```python
from build123d import *

# Parameters (mm, degrees)
F1_DEPTH    = 10
F2_R        = 2.65
F2_R_2      = 2.7
F3_DEPTH    = 10.001
F4_T2_ANGLE = 34.0182957269
F6_DEPTH    = 6
F7_R        = 1.99999
F8_T1_DEPTH = 13.9199888123


# Not quite as in the source:
# - a fillet or chamfer that OpenCascade refuses, or shapes differently, is made with other operations: its cross-section is extruded or revolved along the edge and cut away or added
# - a fillet or chamfer is up to 0.001 mm smaller than in the source, because OpenCascade refuses the exact size


with BuildPart() as f1:
    # F0 (on Top) → F1 (new body)
    with BuildSketch(Plane.XY):
        with BuildLine():
            Line((-33.6606874732, -11.2477834763), (-53.6606874732, -11.1477834763))
            Line((-53.6606874732, -11.1477834763), (-53.7111874732, -21.2477834763))
            Line((-53.7111874732, -21.2477834763), (-41.7113374704, -21.3077827264))
            ThreePointArc((-41.7113374704, -21.3077827264), (-20.1551088941, -33.6039887965), (-10, -56.2477834763))
            Line((-10, -56.2477834763), (0, -56.2477834763))
            ThreePointArc((0, -56.2477834763), (0.8963967025, -47.7664020072), (1.3093095262, -39.2477834763))
            Line((1.3093095262, -39.2477834763), (1.0172378853, -32.2477834763))
            ThreePointArc((1.0172378853, -32.2477834763), (-3.5776423647, -21.3591536143), (-12.6606874732, -13.7978391557))
            Line((-12.6606874732, -13.7978391557), (-21.6606874732, -12.1477834763))
            ThreePointArc((-21.6606874732, -12.1477834763), (-27.6471372828, -11.5171142711), (-33.6606874732, -11.2477834763))
        make_face()
    extrude(amount=F1_DEPTH)

    # F2 (on face) → F3 (cut, through all)
    with BuildSketch(Plane.XY.offset(10)):
        with Locations((-46.6606874732, -17.1477834763)):
            Circle(F2_R)
        with Locations((-16.6606874732, -21.2477834763)):
            Circle(F2_R)
        with Locations((-6.6606874732, -50.2477834763)):
            Circle(F2_R)
        with Locations((-6.6606874732, -30.2477834763)):
            Circle(F2_R_2)
    extrude(amount=-F3_DEPTH, mode=Mode.SUBTRACT)

    # F4: fillet of radius 6 on 1 edges, made by hand

    # F4_s1 → F4_t2 (revolve, cut)
    with BuildSketch(Plane(origin=(-32.1356329931, -81.9445924317, 0), x_dir=(0, 0, 1), z_dir=(-0.3650924394, -0.9309712727, 0))):
        with BuildLine():
            ThreePointArc((0, -18.8349622687), (1.7573593129, -23.0776029558), (6, -24.8349622687))
            Line((6, -24.8349622687), (6, -24.9549622687))
            Line((6, -24.9549622687), (-0.12, -24.9549622687))
            Line((-0.12, -24.9549622687), (-0.12, -18.8349622687))
            Line((-0.12, -18.8349622687), (0, -18.8349622687))
        make_face()
    revolve(axis=Axis((-148.6606874732, -36.2477834763, 0), (0, 0, 1)), revolution_arc=F4_T2_ANGLE, mode=Mode.SUBTRACT)

    # F5 (on face) → F6 (join)
    with BuildSketch(Plane.XY):
        with BuildLine():
            ThreePointArc((-19.6606874732, -34.1590258202), (-19.1967513982, -34.6993177477), (-18.7425076385, -35.2477834763))
            Line((-18.7425076385, -35.2477834763), (-9.6606874732, -35.2477834763))
            Line((-9.6606874732, -35.2477834763), (-9.6606874732, -31.2477834763))
            Line((-9.6606874732, -31.2477834763), (-19.6606874732, -31.2477834763))
            Line((-19.6606874732, -31.2477834763), (-19.6606874732, -34.1590258202))
        make_face()
    extrude(amount=-F6_DEPTH)

    # F7 (radius 2 in the source; OpenCascade refuses exactly that, so slightly less here)
    f7_edges = [f1.edges().sort_by_distance(p)[0] for p in [
        (-19.660687, -31.247783, -3),
        (-9.660687, -31.247783, -3),
        (-9.660687, -35.247783, -3),
    ]]
    fillet(f7_edges, radius=F7_R)

    # F8: fillet of radius 7 on 1 edges, made by hand

    # F8_s2 → F8_t1 (cut)
    with BuildSketch(Plane.XY.offset(-13.9199888123)):
        with BuildLine():
            ThreePointArc((-15.5745121135, -35.2477834763), (-18.3484354275, -34.6747072699), (-20.6681674701, -33.0493118901))
            ThreePointArc((-20.6681674701, -33.0493118901), (-19.6852521083, -34.1309546714), (-18.7425076385, -35.2477834763))
            Line((-18.7425076385, -35.2477834763), (-15.5745121135, -35.2477834763))
        make_face()
    extrude(amount=F8_T1_DEPTH, mode=Mode.SUBTRACT)


solid = f1.part
```
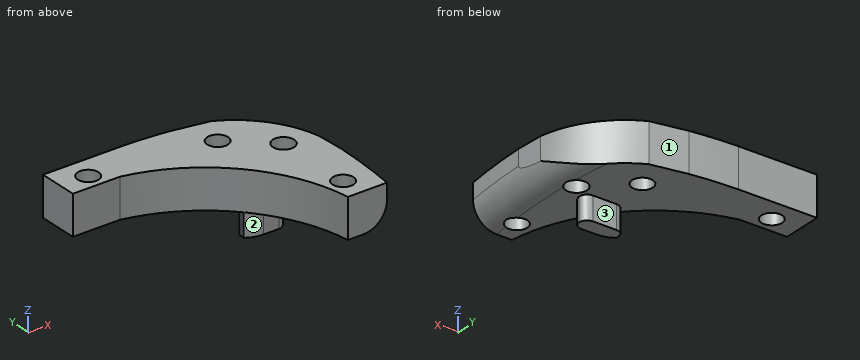
Source: CAD feature listing. Evaluate the final solid. Frame: model axes, mm. Face numbers are marked on the shaded views. A direction names the side the tool comes from. Round coordinates to 2 decimals unless told otherwise and drop trailing zeros. Write each loop counter-clockwise with the first axis right and the second up, starting at its lowest first coordinate (ties: lowest second). Pieces come first, ordered by that corner, then holes. Notation, with made-up numbers: M 36.5,-38.5 L 89.5,-38.5 A19 ccw 89.5,-23.5 Z; hole C 65.5,-29 d3. An arc over 180 degrees is marked long. Use CSV: the item, a comma, the result in double quotes. Start each with the question number.
Q1. Line query: line 1 (Z direction, x = -9, y = -36.5); line 2 (Y direction, x = -5, z = 1.5); line 3 (Y direction, x = -17, z = 1.25). Output: solid intervals per line, ascending. Write a range as from..to.
Q2. Cut plane C-C on x = -36. Output: boundary loops of the cut face in (y, z).
Q3. Cut plane D-D on z = 2. Output: boundary loops of the cut face in (x, y).
Q4. Cut plane B-B on z = 8. Output: boundary loops of the cut face in (x, y), plus the area to 3 significant figures.
Q5. First-contact query: P1, Ø3, axis at x = -14, z = -2.5, coming from the -Y side; P2, Ø0.8, axis at y = -33.5, z = -2, coming from the -X side; P3, Ø8, axis at x = -35.5, z = 8, coming from the -Y side. Flat tips, straight axial feed; report the tip coordinate or a pass-through.
Q6. Access query for the marked faces 1, 2 and 3. Directions: +Z, -Z, +X, -X, +Y, -Y. A direction counts if a zero-diameter tool reaches every point of the face in a straight line with its end or side. Return the directions, or none.
Results found:
1,line 1,"0..10"
1,line 2,"-56.25..-52.31, -48.18..-32.38, -28.12..-19.61"
1,line 3,"-37.56..-23.88, -18.62..-13"
2,outline,"M -22.93,0 L -11.24,0 L -11.24,10 L -22.93,10 Z"
3,outline,"M -53.71,-21.25 L -41.71,-21.31 A40 cw -10,-56.25 L -1.54,-56.25 A148.47 ccw -0.48,-26.87 A25 ccw -12.66,-13.8 L -21.66,-12.15 A100 ccw -33.66,-11.25 L -53.66,-11.15 Z; hole C -46.66,-17.15 d5.3; hole C -16.66,-21.25 d5.3; hole C -6.66,-30.25 d5.4; hole C -6.66,-50.25 d5.3"
4,outline,"M -53.71,-21.25 L -41.71,-21.31 A40 cw -10,-56.25 L 0,-56.25 A150 ccw 1.31,-39.25 L 1.02,-32.25 A25 ccw -12.66,-13.8 L -21.66,-12.15 A100 ccw -33.66,-11.25 L -53.66,-11.15 Z; hole C -46.66,-17.15 d5.3; hole C -16.66,-21.25 d5.3; hole C -6.66,-30.25 d5.4; hole C -6.66,-50.25 d5.3"
4,area,"1,010 mm^2"
5,P1,"y = -35.25"
5,P2,"x = -19.66"
5,P3,"y = -24.91"
6,face 1,"+Z, -Z, +X, +Y"
6,face 2,"-Z, -X, -Y"
6,face 3,"-Z, +X, -X, +Y"
